```python
from build123d import *

# Parameters (mm, degrees)
M2_5_CLEARANCE_HOLE1_D = 3.1


with BuildPart() as part:
    # Sketch1 → Revolve1 (revolve)
    with BuildSketch(Plane(origin=(0, 0, 0), x_dir=(1, 0, 0), z_dir=(0, 1, 0)), mode=Mode.PRIVATE) as revolve1_sk:
        Polygon((1.96, -24), (1.96, 0), (0, 0), (0, 2), (9.525, 2), (9.525, 0), (2.96, 0), (2.96, -24), align=None)
    revolve(revolve1_sk.sketch.rotate(Axis((0, 0, -2), (0, 0, 1)), 180), axis=Axis((0, 0, -2), (0, 0, 1)))

    # M2.5 Clearance Hole1 (through all)
    with Locations(Plane(origin=(0, 2.96, 0), x_dir=(1, 0, 0), z_dir=(0, 1, 0))):
        with Locations((0, -20)):
            Hole(M2_5_CLEARANCE_HOLE1_D / 2)


solid = part.part
```
CAD build for the part. Positions are in the model's coordinates, mm. A direction names the side the tool comes from. Round coordinates to 2 decimals unless told otherwise and drop trailing zeros. Loops run counter-clockwise (first coordinate to the right, second up) from the corner with the lowest first, then second, coordinate; pieces in that order, holes last. Notation, with made-up numbers: M 73,71 L 98,71 A16 cw 98,93 Z; hole C 84.25,-37 d5. An arc over 180 degrees is marked long. Return JSON: item names as keys, results as strings. Group by question number.
(1) Saw through at D-D, the plane z = 14. List the corners of the cut face in (x, y).
(2) Saw through at A-A, the plane x = 0. List the corners of the cut face in (y, z) (3 decimals).
(3) Tool access for faces 4 (the flat face through (-1, 2, 24)), 5 (the cylindrical face through (0.385, -2.935, 12.168)): list every direction of +Z, -Z, +X, -X, +Y, -Y with a clear straight run to the whole face (end or side of a thin tool).
(4) Saw through at B-B, the plane y = 0. List the corners of the cut face in (x, z) (3 decimals), and give its area (3 significant figures).
(5) Saw through at C-C, the plane z = 20. List the corners of the cut face in (x, y).
(6) Drop flat-ended pins along their axis: P1, Ø1.5, axis at y = -1.5, z = 2, coming from the +X side; P2, Ø1.5, axis at y = 0, z = 14.5, coming from the -X side; P3, Ø10, axis at x = -5.5, z = 13, coming from the -Y side. Give the stop position or say it passes through.
(7) Wall check: probe 1 along Y at (x, z) = (0, 5); probe 2 along Z at (x, y) = (0, -1.85); probe 3 along X at (y, z) = (1.5, 5.5). Give the ranges that are in metal, low to high. Write a range as [from, to].
(8) Mould opens along X. For faces 1 (the flat face through (0, 0, -2)), 2 (the cylindrical face through (0.425, 1.913, 11.832)), 3 (the cylindrical face through (2.06, 9.3, -0.99)) say: +X half, -X half, draft (parallel to the pull), parting line (faces both ways), or undercut.
Answer list:
{
 "1": {"outline": "C 0,0 d5.92; hole C 0,0 d3.92"},
 "2": {"outline": "M -9.525,-2 L 9.525,-2 L 9.525,0 L 2.96,0 L 2.96,18.45 L 1.96,18.45 L 1.96,0 L -1.96,0 L -1.96,18.45 L -2.96,18.45 L -2.96,0 L -9.525,0 Z; M -2.96,21.55 L -1.96,21.55 L -1.96,24 L -2.96,24 Z; M 1.96,21.55 L 2.96,21.55 L 2.96,24 L 1.96,24 Z"},
 "3": {"face 4": "+Z, +X, -X, +Y, -Y", "face 5": "+Z"},
 "4": {"outline": "M -9.525,-2 L 9.525,-2 L 9.525,0 L 2.96,0 L 2.96,24 L 1.96,24 L 1.96,0 L -1.96,0 L -1.96,24 L -2.96,24 L -2.96,0 L -9.525,0 Z", "area": "86.1 mm2"},
 "5": {"outline": "M -1.55,-2.52 L -1.55,-1.2 A1.96 cw -1.55,1.2 L -1.55,2.52 A2.96 ccw Z; M 1.55,-2.52 A2.96 ccw 1.55,2.52 L 1.55,1.2 A1.96 cw 1.55,-1.2 Z"},
 "6": {"P1": "x = 2.86", "P2": "x = -2.96", "P3": "y = -2.92"},
 "7": {"probe 1": "[-2.96, -1.96], [1.96, 2.96]", "probe 2": "[-2, 0]", "probe 3": "[-2.55, -1.26], [1.26, 2.55]"},
 "8": {"face 1": "draft", "face 2": "undercut", "face 3": "parting line"}
}
